from build123d import *

# Parameters (mm, degrees)
BOSS_EXTRUDE1_DEPTH = 13.35
SKETCH3_R           = 9
CUT_EXTRUDE1_DEPTH  = 23
SKETCH4_R           = 11.5
CUT_EXTRUDE3_DEPTH  = 35.7
SKETCH7_R           = 9
CUT_EXTRUDE9_DEPTH  = 49.85
BOSS_EXTRUDE2_START = 25
SKETCH8_R           = 12.5
SKETCH8_R_2         = 9
BOSS_EXTRUDE2_DEPTH = 25


with BuildPart() as part:
    # Sketch2 → Boss-Extrude1 (new, symmetric)
    with BuildSketch(Plane.XY):
        Polygon((0, -13.35), (13.35, -13.35), (13.35, 63.2), (-26.7, 63.2), (-26.7, 36.5), (-13.35, 36.5), (-13.35, -13.35), align=None)
    extrude(amount=BOSS_EXTRUDE1_DEPTH, both=True)

    # Sketch3 → Cut-Extrude1 (cut)
    with BuildSketch(Plane.XY.offset(13.35)):
        Circle(SKETCH3_R)
    extrude(amount=-CUT_EXTRUDE1_DEPTH, mode=Mode.SUBTRACT)

    # Sketch4 → Cut-Extrude3 (cut)
    with BuildSketch(Plane.ZY.offset(26.7)):
        with Locations((0, 49.85)):
            Circle(SKETCH4_R)
    extrude(amount=-CUT_EXTRUDE3_DEPTH, mode=Mode.SUBTRACT)

    # Sketch7 → Cut-Extrude9 (cut)
    with BuildSketch(Plane(origin=(0, 0, 0), x_dir=(1, 0, 0), z_dir=(0, 1, 0))):
        Circle(SKETCH7_R)
    extrude(amount=CUT_EXTRUDE9_DEPTH, mode=Mode.SUBTRACT)

    # Sketch8 → Boss-Extrude2 (add)
    with BuildSketch(Plane.XY.offset(13.35).offset(BOSS_EXTRUDE2_START)):
        Circle(SKETCH8_R)
        Circle(SKETCH8_R_2, mode=Mode.SUBTRACT)
    extrude(amount=-BOSS_EXTRUDE2_DEPTH)


solid = part.part
For this review, take the finished solid that the model builds, in its own axes (mm). A direction names the side the tool comes from. Give positions to 0.01 mm unless a question says otherwise; leave off trailing zeros. Order: outer loops, then holes, each group sorted by start corner. A loop starts at its lowest first (then second) coordinate and runs counter-clockwise, first axis right, second up. Notation, with made-up numbers: (14.5, -20.5) -> (29.5, -20.5) arc R27 ccw to (29.5, 0.5) -> close; hole circle Ø9 at (49, 88). An arc over 180 degrees is marked (long way). Write item = value, one per line.
1) We need section D-D, the plane y = 11. Give the boundary of the cut face in (x, z), and give its area (3 significant figures).
Findings:
outline = (-13.35, -13.35) -> (13.35, -13.35) -> (13.35, 13.35) -> (5.94, 13.35) -> (5.94, 38.35) -> (-5.94, 38.35) -> (-5.94, 13.35) -> (-13.35, 13.35) -> close; hole circle Ø18 at (0, 0)
area = 755 mm^2
2) Insertion check: pin 1 (13.5 mm diameter, centred on y = 18, z = 5, fed in from -X); pin 2 (2 mm diameter, centred on y = 53.5, z = -6.5, fed in from -X); pin 3 (8 mm diameter, centred on y = -2.5, z = 23.5, fed in from -X). Each pin has a flat end and moves straight along its axis. Give the tip position at first contact, or say it passes through.
Findings:
pin_1 = -13.35
pin_2 = 9
pin_3 = -12.5
3) We need section C-C, the plane z = 31. Give the boundary of the cut face in (x, y).
Findings:
outline = circle Ø25 at (0, 0); hole circle Ø18 at (0, 0)
4) Draft analysis for pull direction Y (two halves, no side actions). For faces 1 (the face through (13.35, 24, 0)), 2 (the face through (11.923, 3.755, 26.025)), 3 (the face through (9, 50, 0)), state which applies: pulls with the +Y half, pulls with the -Y half, needs draft (parallel to the pull), parting line crosses it, or undercut.
Findings:
face_1 = needs draft
face_2 = parting line crosses it
face_3 = undercut
5) To check wall thickness, follow L1, parallel to X at y = 11, z = 0; L2, parallel to Y at x = 0, z = 12.5; L3, parallel to Z at x = 0, y = 11.5. State the ranges of each line that lie inside material, in increasing order. Write a range as from..to.
Findings:
L1 = -13.35..-9, 9..13.35
L2 = -13.35..-9, 9..63.2
L3 = -13.35..-9, 9..38.35
6) We need section B-B, the plane x = -19.5. Give the boundary of the cut face in (y, z).
Findings:
outline = (36.5, -13.35) -> (63.2, -13.35) -> (63.2, 13.35) -> (36.5, 13.35) -> close; hole circle Ø23 at (49.85, 0)
7) For faces 4 (the face through (-6.633, 21.047, -6.083)), 5 (the face through (-1.951, -8.786, 14.686)), 6 (the face through (-20, 36.5, 0)), list the 3-axis set-ups (+Z, -Z, +X, -X, +Y, -Y) from which the entire face can be reached by the end or side of a thin tool; tool diameter is ignored.
Findings:
face_4 = none
face_5 = +Z
face_6 = +Z, -Z, -X, -Y
